The listing builds one solid part. Answer for the finished solid, in the listing's coordinates (mm). Face numbers are marked on the shaded views. A direction names the side the tool comes from. Coordinates: 2 decimals unless noted, no trailing zeros. Order: outer loops, then holes, each group sorted by start corner. A loop starts at its lowest first (then second) coordinate and runs counter-clockwise, first axis right, second up. Notation, with made-up numbers: (83.25, 7.5) -> (88.25, 7.5) arc R21 ccw to (88.25, 14.5) -> close; hole circle Ø7 at (23, 4). An arc over 180 degrees is marked (long way). Answer in a Markdown table with one row per item.
```python
from build123d import *

# Parameters (mm, degrees)
SKETCH2_W           = 42.3
SKETCH2_H           = 42.3
BOSS_EXTRUDE1_DEPTH = 13
SKETCH3_R           = 11
CUT_EXTRUDE1_DEPTH  = 14
SKETCH4_R           = 1.75
CUT_EXTRUDE2_DEPTH  = 14
SKETCH5_R           = 29.910616844
SKETCH5_R_2         = 27
CUT_EXTRUDE4_DEPTH  = 14
CUT_EXTRUDE5_DEPTH  = 11
SKETCH7_R           = 16
BOSS_EXTRUDE2_DEPTH = 6
SKETCH8_R           = 0.9
BOSS_EXTRUDE3_DEPTH = 2.5
CHAMFER1_SIZE       = 0.3
CHAMFER2_SIZE       = 0.3
SKETCH9_R           = 12
CUT_EXTRUDE6_DEPTH  = 3
CHAMFER4_SIZE       = 0.5


with BuildPart() as part:
    # Sketch2 → Boss-Extrude1 (new body)
    with BuildSketch(Plane(origin=(0, 0, 0), x_dir=(1, 0, 0), z_dir=(0, 1, 0))):
        Rectangle(SKETCH2_W, SKETCH2_H)
    extrude(amount=BOSS_EXTRUDE1_DEPTH)

    # Sketch3 → Cut-Extrude1 (cut, through all)
    with BuildSketch(Plane(origin=(0, 13, 0), x_dir=(1, 0, 0), z_dir=(0, 1, 0))):
        Circle(SKETCH3_R)
    extrude(amount=-CUT_EXTRUDE1_DEPTH, mode=Mode.SUBTRACT)

    # Sketch4 → Cut-Extrude2 (cut, through all)
    with BuildSketch(Plane(origin=(0, 13, 0), x_dir=(1, 0, 0), z_dir=(0, 1, 0))):
        with Locations((-15.5, 15.5)):
            Circle(SKETCH4_R)
        with Locations((15.5, 15.5)):
            Circle(SKETCH4_R)
        with Locations((15.5, -15.5)):
            Circle(SKETCH4_R)
        with Locations((-15.5, -15.5)):
            Circle(SKETCH4_R)
    extrude(amount=-CUT_EXTRUDE2_DEPTH, mode=Mode.SUBTRACT)

    # Sketch5 → Cut-Extrude4 (cut, through all)
    with BuildSketch(Plane(origin=(0, 13, 0), x_dir=(1, 0, 0), z_dir=(0, 1, 0))):
        Circle(SKETCH5_R)
        Circle(SKETCH5_R_2, mode=Mode.SUBTRACT)
    extrude(amount=-CUT_EXTRUDE4_DEPTH, mode=Mode.SUBTRACT)

    # Sketch6 → Cut-Extrude5 (cut)
    with BuildSketch(Plane(origin=(0, 13, 0), x_dir=(1, 0, 0), z_dir=(0, 1, 0))):
        with BuildLine():
            Line((-21.15, 4.305844123), (-12.727922061, 12.727922061))
            ThreePointArc((-12.727922061, 12.727922061), (12.727922061, 12.727922061), (12.727922061, -12.727922061))
            Line((12.727922061, -12.727922061), (4.305844123, -21.15))
            Line((4.305844123, -21.15), (-5.593650814, -21.15))
            Line((-5.593650814, -21.15), (-2.296546247, -17.852895433))
            ThreePointArc((-2.296546247, -17.852895433), (-12.727922061, -12.727922061), (-17.852895433, -2.296546247))
            Line((-17.852895433, -2.296546247), (-21.15, -5.593650814))
            Line((-21.15, -5.593650814), (-21.15, 4.305844123))
        make_face()
    extrude(amount=-CUT_EXTRUDE5_DEPTH, mode=Mode.SUBTRACT)

    # Sketch7 → Boss-Extrude2 (add)
    with BuildSketch(Plane(origin=(0, 2, 0), x_dir=(1, 0, 0), z_dir=(0, 1, 0))):
        with BuildLine():
            Line((-21.15, 4.305844123), (-21.15, -5.593650814))
            Line((-21.15, -5.593650814), (-17.852895433, -2.296546247))
            ThreePointArc((-17.852895433, -2.296546247), (-12.727922061, -12.727922061), (-2.296546247, -17.852895433))
            Line((-2.296546247, -17.852895433), (-5.593650814, -21.15))
            Line((-5.593650814, -21.15), (4.305844123, -21.15))
            Line((4.305844123, -21.15), (12.727922061, -12.727922061))
            ThreePointArc((12.727922061, -12.727922061), (12.727922061, 12.727922061), (-12.727922061, 12.727922061))
            Line((-12.727922061, 12.727922061), (-21.15, 4.305844123))
        make_face()
        Circle(SKETCH7_R, mode=Mode.SUBTRACT)
    extrude(amount=BOSS_EXTRUDE2_DEPTH)

    # Sketch8 → Boss-Extrude3 (add)
    with BuildSketch(Plane(origin=(0, 13, 0), x_dir=(1, 0, 0), z_dir=(0, 1, 0))):
        with Locations((12.671572875, 18.328427125)):
            Circle(SKETCH8_R)
        with Locations((18.328427125, 12.671572875)):
            Circle(SKETCH8_R)
        with Locations((-12.671572875, -18.328427125)):
            Circle(SKETCH8_R)
        with Locations((-18.328427125, -12.671572875)):
            Circle(SKETCH8_R)
    extrude(amount=BOSS_EXTRUDE3_DEPTH)

    # Chamfer1
    chamfer1_edges = [part.edges().sort_by_distance(p)[0] for p in [
        (11.771572875, 15.5, -18.328427125),
        (17.428427125, 15.5, -12.671572875),
        (-13.571572875, 15.5, 18.328427125),
        (-19.228427125, 15.5, 12.671572875),
    ]]
    chamfer(chamfer1_edges, length=CHAMFER1_SIZE)

    # Chamfer2
    chamfer2_edges = [part.edges().sort_by_distance(p)[0] for p in [
        (11.771572875, 13, -18.328427125),
        (17.428427125, 13, -12.671572875),
        (-13.571572875, 13, 18.328427125),
        (-19.228427125, 13, 12.671572875),
    ]]
    chamfer(chamfer2_edges, length=CHAMFER2_SIZE)

    # Sketch9 → Cut-Extrude6 (cut, through all)
    with BuildSketch(Plane(origin=(0, 2, 0), x_dir=(1, 0, 0), z_dir=(0, 1, 0))):
        Circle(SKETCH9_R)
    extrude(amount=-CUT_EXTRUDE6_DEPTH, mode=Mode.SUBTRACT)

    # Chamfer4
    chamfer4_edges = [part.edges().sort_by_distance(p)[0] for p in [
        (-17.25, 0, 15.5),
        (13.75, 0, 15.5),
        (13.75, 0, -15.5),
        (-17.25, 0, -15.5),
    ]]
    chamfer(chamfer4_edges, length=CHAMFER4_SIZE)


solid = part.part
```
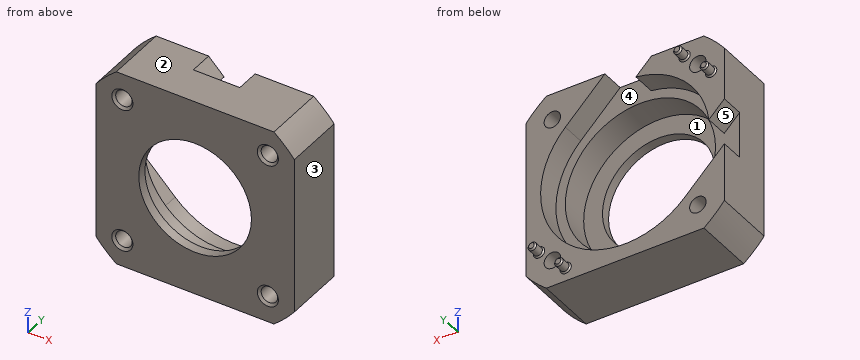
(1) For a pull along X with two mould halves and no side action, classify the marked faces 3, 4 and 5 as released by +X, released by -X, zero draft, split by the parting line, or undercut.
Check values:
| item | result |
|---|---|
| face 3 | released by +X |
| face 4 | undercut |
| face 5 | released by -X |
(2) A cutting plane is placed at B-B, the plane x = 0. Determine the outline of the cut face in (y, z), then the cut area to 3 significant figures.
Check values:
| item | result |
|---|---|
| outline | (0, -21.15) -> (13, -21.15) -> (13, -18) -> (8, -18) -> (8, -16) -> (2, -16) -> (2, -12) -> (0, -12) -> close; (0, 12) -> (2, 12) -> (2, 16) -> (8, 16) -> (8, 21.15) -> (0, 21.15) -> close |
| area | 114 mm² |
(3) Which of the six approach directions +Z, -Z, +X, -X, +Y, -Y give full straight-line access (tool end or side, diameter ignored) to the marked faces 1 and 2?
Check values:
| item | result |
|---|---|
| face 1 | +Y |
| face 2 | +Z, +X, -X, +Y, -Y |
(4) Find the intervals of material crossed by line 1 along Z through (x, y) = (0, 1.4); line 2 along X through (y, z) = (4.15, 0), in increasing order. Write a range as from..to.
Check values:
| item | result |
|---|---|
| line 1 | -21.15..-12, 12..21.15 |
| line 2 | -21.15..-16, 16..21.15 |
(5) A cutting plane is placed at C-C, the plane z = 0. Determine the outline of the cut face in (x, y), then the cut area to 3 significant figures.
Check values:
| item | result |
|---|---|
| outline | (-21.15, 0) -> (-12, 0) -> (-12, 2) -> (-16, 2) -> (-16, 8) -> (-21.15, 8) -> close; (12, 0) -> (21.15, 0) -> (21.15, 13) -> (18, 13) -> (18, 8) -> (16, 8) -> (16, 2) -> (12, 2) -> close |
| area | 114 mm² |
(6) Flat-ended cylindrical pins translate along their axes: pin 1 (20.5 mm diameter, centred on x = -14, z = 12.5, fed in from +Y); pin 2 (21 mm diameter, centred on x = 7, z = 0, fed in from +Y); pin 3 (3 mm diameter, centred on x = -15.5, z = -15.5, fed in from -Y); pin 4 (3 mm diameter, centred on x = 8, z = 9, fed in from +Y). Find the tip coordinate at first contact, or state that the pin passes through.
Check values:
| item | result |
|---|---|
| pin 1 | y = 15.5 |
| pin 2 | y = 8 |
| pin 3 | through |
| pin 4 | y = 2 |
(7) A cutting plane is placed at D-D, the plane z = 15.5. Determine the outline of the cut face in (x, y).
Check values:
| item | result |
|---|---|
| outline | (-21.15, 0) -> (-17.75, 0) -> (-17.25, 0.5) -> (-17.25, 13) -> (-21.15, 13) -> close; (-13.75, 0.5) -> (-13.25, 0) -> (13.25, 0) -> (13.75, 0.5) -> (13.75, 13) -> (9.96, 13) -> (9.96, 8) -> (3.97, 8) -> (3.97, 2) -> (-3.97, 2) -> (-3.97, 8) -> (-9.15, 8) -> (-9.15, 13) -> (-13.75, 13) -> close; (17.25, 0.5) -> (17.75, 0) -> (21.15, 0) -> (21.15, 13) -> (17.25, 13) -> close |
(8) A cutting plane is placed at A-A, the plane y = 3.25. Determine the outline of the cut face in (x, z).
Check values:
| item | result |
|---|---|
| outline | (-21.15, -16.78) arc R27 ccw to (-16.78, -21.15) -> (16.78, -21.15) arc R27 ccw to (21.15, -16.78) -> (21.15, 16.78) arc R27 ccw to (16.78, 21.15) -> (-16.78, 21.15) arc R27 ccw to (-21.15, 16.78) -> close; hole circle Ø3.5 at (-15.5, -15.5); hole circle Ø3.5 at (-15.5, 15.5); hole circle Ø32 at (0, 0); hole circle Ø3.5 at (15.5, -15.5); hole circle Ø3.5 at (15.5, 15.5) |
